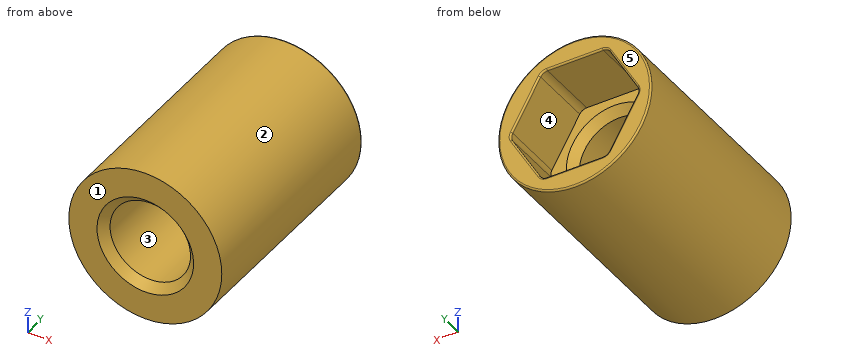
```python
from build123d import *

# Parameters (mm, degrees)
SKETCH1_R           = 4.75
SKETCH1_R_2         = 2.5
BOSS_EXTRUDE1_DEPTH = 14
CUT_EXTRUDE1_DEPTH  = 4
FILLET1_R           = 0.5
CHAMFER1_SIZE       = 0.5
FILLET2_R           = 0.1


with BuildPart() as part:
    # Sketch1 → Boss-Extrude1 (new body)
    with BuildSketch(Plane(origin=(0, 0, 0), x_dir=(1, 0, 0), z_dir=(0, 1, 0))):
        with Locations(Location((0, 0, 0), (0, 0, 270))):
            Circle(SKETCH1_R)
        with Locations(Location((0, 0, 0), (0, 0, 270))):
            Circle(SKETCH1_R_2, mode=Mode.SUBTRACT)
    extrude(amount=BOSS_EXTRUDE1_DEPTH)

    # Sketch2 → Cut-Extrude1 (cut)
    with BuildSketch(Plane(origin=(0, 14, 0), x_dir=(1, 0, 0), z_dir=(0, 1, 0))):
        Polygon((4.041451884, 0), (2.020725942, 3.5), (-2.020725942, 3.5), (-4.041451884, 0), (-2.020725942, -3.5), (2.020725942, -3.5), align=None)
    extrude(amount=-CUT_EXTRUDE1_DEPTH, mode=Mode.SUBTRACT)

    # Fillet1
    fillet1_edges = [part.edges().sort_by_distance(p)[0] for p in [
        (4.041451884, 12, 0),
        (2.020725942, 12, 3.5),
        (-2.020725942, 12, 3.5),
        (-4.041451884, 12, 0),
        (-2.020725942, 12, -3.5),
        (2.020725942, 12, -3.5),
    ]]
    fillet(fillet1_edges, radius=FILLET1_R)

    # Chamfer1
    chamfer1_edges = [part.edges().sort_by_distance(p)[0] for p in [
        (0, 10, -2.5),
        (0, 0, -2.5),
    ]]
    chamfer(chamfer1_edges, length=CHAMFER1_SIZE)

    # Fillet2
    fillet2_edges = [part.edges().sort_by_distance(p)[0] for p in [
        (3.031088913, 14, 1.75),
        (0, 14, 3.5),
        (-3.031088913, 14, 1.75),
        (0, 14, -4.75),
        (-3.031088913, 14, -1.75),
        (3.031088913, 14, -1.75),
        (0, 14, -3.5),
        (1.982050808, 14, 3.433012702),
        (-1.982050808, 14, 3.433012702),
        (-3.964101615, 14, 0),
        (3.964101615, 14, 0),
        (1.982050808, 14, -3.433012702),
        (-1.982050808, 14, -3.433012702),
    ]]
    fillet(fillet2_edges, radius=FILLET2_R)


solid = part.part
```
Build history of the part. All positions in model axes, mm. Face numbers are marked on the shaded views. A direction names the side the tool comes from. Round coordinates to 2 decimals unless told otherwise and drop trailing zeros. Write each loop counter-clockwise with the first axis right and the second up, starting at its lowest first coordinate (ties: lowest second). Pieces come first, ordered by that corner, then holes.
1) Band-saw the part on D-D, the plane y = 3.75. List the corners of the cut face in (x, z), and give its area (3 significant figures).
2) Band-saw the part on B-B, the plane z = 0. List the corners of the cut face in (x, y).
3) Pin check, flat tips, straight feed: pin 1 (1.5 mm diameter, centred on x = -1.5, y = 10, fed in from -Z); pin 2 (1 mm diameter, centred on x = -3, z = 0, fed in from +Y); pin 3 (1 mm diameter, centred on y = 12.5, z = 1, fed in from +X); pin 4 (3 mm diameter, centred on x = 0, z = 0, fed in from -Y). Stop position of each tip, or through.
4) Band-saw the part on A-A, the plane x = 0. List the corners of the cut face in (y, z), and give its area (3 significant figures).
5) Band-saw the part on C-C, the plane y = 12.25. List the corners of the cut face in (x, z).
6) 3-axis set-ups, long thin cutter, end or side, ignore diameter. For the marked faces 4 and 5: which of +Z, -Z, +X, -X, +Y, -Y reach the whole face in a straight line?
7) Mould opens along Z. For the marked faces 1, 2 and 3 say: +Z half, -Z half, draft (parallel to the pull), parting line (faces both ways), or undercut.
8) Drill centre lines: probe 1 along X at (y, z) = (13.5, 0); probe 2 along X at (y, z) = (6.5, 0); probe 3 along Z at (x, y) = (0.75, 2.75). Where is each one in solid material? Low to high.
Ans:
1. outline: circle Ø9.5 at (0, 0); hole circle Ø5 at (0, 0)
1. area: 51.2 mm2
2. outline: (-4.75, 0) - (-3, 0) - (-2.5, 0.5) - (-2.5, 9.5) - (-3, 10) - (-3.96, 10) - (-3.96, 13.9) arc R0.1 ccw to (-4.06, 14) - (-4.65, 14) arc R0.1 ccw to (-4.75, 13.9) - close; (2.5, 0.5) - (3, 0) - (4.75, 0) - (4.75, 13.9) arc R0.1 ccw to (4.65, 14) - (4.06, 14) arc R0.1 ccw to (3.96, 13.9) - (3.96, 10) - (3, 10) - (2.5, 9.5) - close
3. pin 1: stops at z = -4.69
3. pin 2: stops at y = 10
3. pin 3: stops at x = 4.72
3. pin 4: passes through
4. outline: (0, -4.75) - (13.9, -4.75) arc R0.1 ccw to (14, -4.65) - (14, -3.6) arc R0.1 ccw to (13.9, -3.5) - (10, -3.5) - (10, -3) - (9.5, -2.5) - (0.5, -2.5) - (0, -3) - close; (0, 3) - (0.5, 2.5) - (9.5, 2.5) - (10, 3) - (10, 3.5) - (13.9, 3.5) arc R0.1 ccw to (14, 3.6) - (14, 4.65) arc R0.1 ccw to (13.9, 4.75) - (0, 4.75) - close
4. area: 54.5 mm2
5. outline: circle Ø9.5 at (0, 0); hole (-3.9, -0.25) - (-2.17, -3.25) arc R0.5 ccw to (-1.73, -3.5) - (1.73, -3.5) arc R0.5 ccw to (2.17, -3.25) - (3.9, -0.25) arc R0.5 ccw to (3.9, 0.25) - (2.17, 3.25) arc R0.5 ccw to (1.73, 3.5) - (-1.73, 3.5) arc R0.5 ccw to (-2.17, 3.25) - (-3.9, 0.25) arc R0.5 ccw to start
6. face 4: +Y
6. face 5: +Z, -Z, +X, -X, +Y
7. face 1: draft
7. face 2: parting line
7. face 3: undercut
8. probe 1: x = -4.75 to -3.96, 3.96 to 4.75
8. probe 2: x = -4.75 to -2.5, 2.5 to 4.75
8. probe 3: z = -4.69 to -2.38, 2.38 to 4.69
